Job drawing, mm, ordinate dimensions from the low corner. One solid piece. A direction names the side the tool comes from. Round coordinates to 2 decimals unless told otherwise and drop trailing zeros. Loops run counter-clockwise (first coordinate to the right, second up) from the corner with the lowest first, then second, coordinate; pieces in that order, holes last. Notation, with made-up numbers: M 75.25,43 L 124.25,43 A17 cw 124.25,73 Z; hole C 82,-16.5 d4. An arc over 180 degrees is marked long. Use a Markdown table: item, result. Add a question column.
(1) Flat gauge pins, fed straight in: P1, Ø4, axis at x = 9, z = 8.5, coming from the -Y side; P2, Ø3, axis at x = 12, y = 3.5, coming from the -Z side; P3, Ø6.5, axis at x = 7.875, z = 7.875, coming from the +Y side. Where does each tip first touch, or does it go through?
(2) Band-saw the part on C-C, the plane x = 14.75. Write the cut outline in (y, z).
(3) Which spindle directions (+Z, -Z, +X, -X, +Y, -Y) get a long thin tool onto all of the face, cutting with end or side? Do the marked faces 1 and 2. Say none if no direction does.
(4) Band-saw the part on A-A, the plane y = 6.75. Write the cut outline in (x, z) (3 decimals), and give its area (3 significant figures).
(5) Band-saw the part on D-D, the plane y = 3.5. Write the cut outline in (x, z) (3 decimals), and give its area (3 significant figures).
(6) Two-plate mould, pull along Z, no slides. Class the marked faces 3, 4, 5 and 6: released by +Z, released by -Z, zero draft, split by the parting line, or undercut.
(7) Wall check: L1, parallel to X at y = 0.5, z = 4.5; L2, parallel to X at y = 5.5, z = 8.25; L3, parallel to Z at x = 9.5, y = 2.25. Give the ranges that are in metal, low to high.
(8) Band-saw the part on B-B, the plane z = 2.5. Write the cut outline in (x, y), and give its area (3 significant figures).
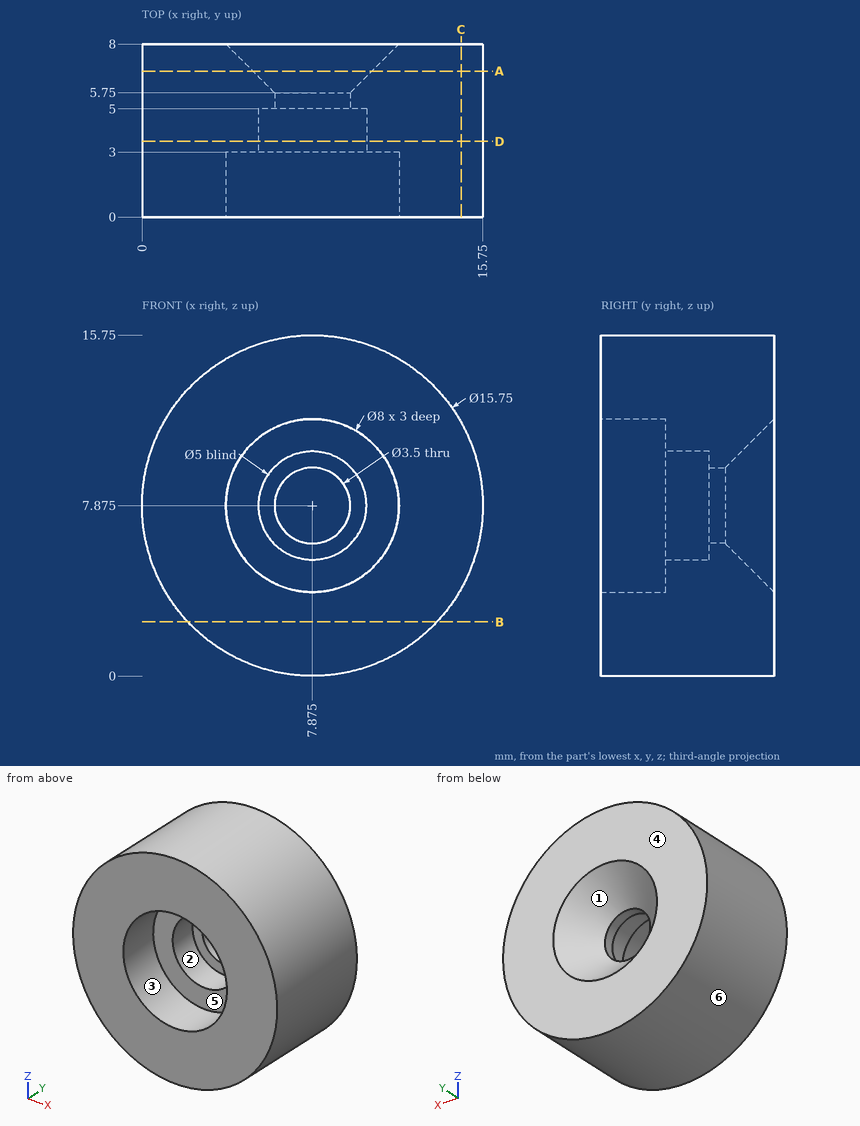
Return value:
| question | item | result |
|---|---|---|
| 1 | P1 | y = 3 |
| 1 | P2 | z = 0.45 |
| 1 | P3 | y = 7.25 |
| 2 | outline | M 0,4.03 L 8,4.03 L 8,11.72 L 0,11.72 Z |
| 3 | face 1 | +Y |
| 3 | face 2 | -Y |
| 4 | outline | C 7.875,7.875 d15.75; hole C 7.875,7.875 d5.5 |
| 4 | area | 171 mm^2 |
| 5 | outline | C 7.875,7.875 d15.75; hole C 7.875,7.875 d5 |
| 5 | area | 175 mm^2 |
| 6 | face 3 | undercut |
| 6 | face 4 | zero draft |
| 6 | face 5 | undercut |
| 6 | face 6 | split by the parting line |
| 7 | L1 | 0.76 to 5.73, 10.02 to 14.99 |
| 7 | L2 | 0.01 to 6.17, 9.58 to 15.74 |
| 7 | L3 | 0.17 to 4.22, 11.53 to 15.58 |
| 8 | outline | M 2.12,0 L 13.63,0 L 13.63,8 L 2.12,8 Z |
| 8 | area | 92.1 mm^2 |
